Geometry: final body of the model. Coordinates: model frame, mm. A direction names the side the tool comes from. Round coordinates to 2 decimals unless told otherwise and drop trailing zeros. Write each loop counter-clockwise with the first axis right and the second up, starting at its lowest first coordinate (ties: lowest second). Pieces come first, ordered by that corner, then holes. Notation, with made-up numbers: (74.5, 1.25) - (97.5, 1.25) arc R14 cw to (97.5, 19.25) - close; hole circle Ø9 at (-35.75, 57). An arc over 180 degrees is marked (long way). Write each question's results on one line, items separated by ' | '.
Autodesk Inventor part; units mm, degrees
ref_plane "YZ Plane" through (0, 0, 0) normal (1, 0, 0) x (0, 1, 0)
ref_plane "XZ Plane" through (0, 0, 0) normal (0, 1, 0) x (-1, 0, 0)
sketch "スケッチ7" plane through (0, 0, 0) normal (0, 0, 1) x (1, 0, 0)
  circle A0 centre (0, 0) radius 25
  dimension "d32" = 50
ref_plane "作業平面7" through (0, 0, 15) normal (0, 0, 1) x (1, 0, 0)
sketch "スケッチ8" plane through (0, 0, 15) normal (0, 0, 1) x (1, 0, 0)
  circle A0 centre (0, 0) radius 22.5
  dimension "d34" = 45
loft "ロフト2" add profiles "スケッチ7", "スケッチ8"
sketch "スケッチ5" plane through (0, 0, 15) normal (0, 0, 1) x (1, 0, 0)
  point P0 (0, 0)
  point P1 (0, 0)
hole "穴1" at (0, 0, 15) direction (0, 0, -1) diameter 8 end through all
sketch "スケッチ6" plane through (0, 0, 15) normal (0, 0, 1) x (1, 0, 0)
  point P0 (0, 0)
  point P1 (15, 0)
  point P2 (0, 15)
  point P3 (-15, 0)
  point P4 (0, -15)
  point P5 (0, 0)
  dimension "d21" = 360
  dimension "d23" = 30
hole "穴2" at (15, 0, 15) at (0, 15, 15) at (-15, 0, 15) at (0, -15, 15) direction (0, 0, -1) diameter 3.4587 depth 10.8 tip angle 118
properties part number "Stator_N5065"
Q1. Ray query, line 1 along X through (y, z) = (0, 11.25) (3 decimals); line 2 along Y through (x, z) = (0, 12.75) (3 decimals); line 3 along Y through (x, z) = (0, 7). Return the intervals inside material, ascending.
Answer block:
line 1: -23.125 to -16.729, -13.271 to -4, 4 to 13.271, 16.729 to 23.125 | line 2: -22.875 to -16.729, -13.271 to -4, 4 to 13.271, 16.729 to 22.875 | line 3: -23.83 to -16.73, -13.27 to -4, 4 to 13.27, 16.73 to 23.83
Q2. Access query for faces 4 (the cylindrical face through (3.905, 0.867, 7.395)), 5 (the cylindrical face through (-13.31, 0.37, 9.52)). Directions: +Z, -Z, +X, -X, +Y, -Y. A direction counts if a zero-diameter tool reaches every point of the face in a straight line with its end or side. Return the directions, or none.
Answer block:
face 4: +Z, -Z | face 5: +Z
Q3. Pin query (flat end, axial travel): pin 1 (1 mm diameter, centred on y = -14, z = 11.5, fed in from -X); pin 2 (6 mm diameter, centred on y = 6, z = 5, fed in from -X); pin 3 (1 mm diameter, centred on y = 12, z = 10.5, fed in from +X). Return the tip coordinate at first contact, or that it passes through.
Answer block:
pin 1: x = -18.74 | pin 2: x = -24.21 | pin 3: x = 20.22
Q4. Mould query, pull axis X, two halves, no side actions, for faces 1 (the cylindrical face through (0.66, -16.6, 9.52)), 2 (the flat face through (0, -5, 0)), 3 (the conical face through (21.44, 8.89, 10.73)). Classes: pulls with the +X half, pulls with the -X half, needs draft (parallel to the pull), parting line crosses it, or undercut.
Answer block:
face 1: undercut | face 2: needs draft | face 3: parting line crosses it
Q5. Section query C-C, the plane z = 7.75. Return loops of the section in (x, y), plus the area to 3 significant figures.
Answer block:
outline: circle Ø47.42 at (0, 0); hole circle Ø3.46 at (-15, 0); hole circle Ø8 at (0, 0); hole circle Ø3.46 at (0, -15); hole circle Ø3.46 at (0, 15); hole circle Ø3.46 at (15, 0) | area: 1,680 mm2
Q6. Section query B-B, the plane z = 1.75. Return loops of the section in (x, y).
Answer block:
outline: circle Ø49.42 at (0, 0); hole circle Ø8 at (0, 0)
Q7. Section query A-A, the plane z = 11. Return loops of the section in (x, y).
Answer block:
outline: circle Ø46.33 at (0, 0); hole circle Ø3.46 at (-15, 0); hole circle Ø8 at (0, 0); hole circle Ø3.46 at (0, -15); hole circle Ø3.46 at (0, 15); hole circle Ø3.46 at (15, 0)
